Geometry check sheet. Reference: the model listing, model coordinates, mm. Give positions to 0.01 mm unless a question says otherwise; leave off trailing zeros. Loops run counter-clockwise (first coordinate to the right, second up) from the corner with the lowest first, then second, coordinate; pieces in that order, holes last. Notation, with made-up numbers: (45.5, -12.5) -> (79.5, -12.5) arc R20 cw to (79.5, 19.5) -> close; hole circle Ø7 at (33.5, 83). An arc over 180 degrees is marked (long way). Write item = value, one per line. Start each with the question number.
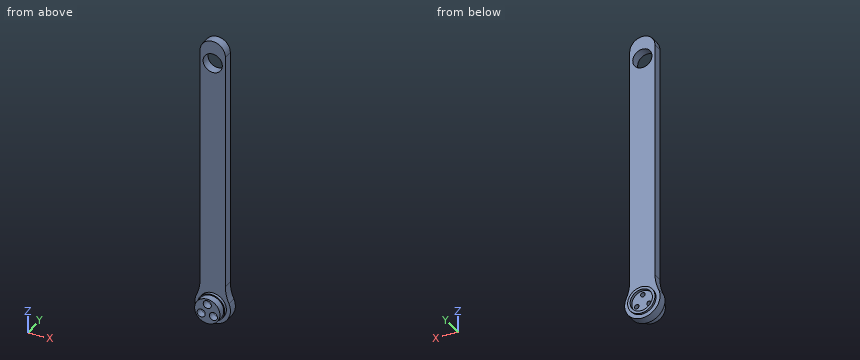
```python
from build123d import *
from build123d.topology import SkipClean

# Parameters (mm, degrees)
EXTRUDE_1_DEPTH              = 9
SKETCH_3_R                   = 13.5
EXTRUDE_2_DEPTH              = 2
SKETCH_4_R                   = 13.5
EXTRUDE_3_DEPTH              = 3
SKETCH_5_R                   = 9.5
CUT_EXTRUDE_2_DEPTH          = 274.324898244
HOLE_WIZARD_M4_1_D           = 4.5
HOLE_WIZARD_M4_1_CBORE_D     = 8
HOLE_WIZARD_M4_1_CBORE_DEPTH = 4.4
PATTERN_CIRCULAR_1_COUNT     = 3
SKETCH_11_R                  = 12.5
SKETCH_11_R_2                = 4
EXTRUDE_4_DEPTH              = 7
SKETCH_13_R                  = 11
CUT_EXTRUDE_3_DEPTH          = 3
FILLET_1_R                   = 40


with BuildPart() as part:
    # Sketch 1 → Extrude 1 (new body)
    with BuildSketch(Plane(origin=(0, 0, 0), x_dir=(1, 0, 0), z_dir=(0, 1, 0))):
        with BuildLine():
            Line((-12.5, -260), (-12.5, -12.247448714))
            ThreePointArc((-12.5, -12.247448714), (0, 17.5), (12.5, -12.247448714))
            Line((12.5, -12.247448714), (12.5, -260))
            ThreePointArc((12.5, -260), (0, -272.5), (-12.5, -260))
        make_face()
    extrude(amount=EXTRUDE_1_DEPTH)

    # Sketch 3 → Extrude 2 (add)
    with BuildSketch(Plane(origin=(0, 9, 0), x_dir=(1, 0, 0), z_dir=(0, 1, 0))):
        with Locations(Location((0, 0, 0), (0, 0, 270))):
            Circle(SKETCH_3_R)
    extrude(amount=EXTRUDE_2_DEPTH)

    # Sketch 4 → Extrude 3 (add)
    with BuildSketch(Plane.XZ):
        with Locations(Location((0, 0, 0), (0, 0, 90))):
            Circle(SKETCH_4_R)
    extrude(amount=EXTRUDE_3_DEPTH)

    # Sketch 5 → Cut-Extrude 2 (cut, through all)
    with BuildSketch(Plane(origin=(0, 9, 0), x_dir=(1, 0, 0), z_dir=(0, 1, 0))):
        with Locations(Location((0, -250, 0), (0, 0, 270))):
            Circle(SKETCH_5_R)
    extrude(amount=-CUT_EXTRUDE_2_DEPTH, mode=Mode.SUBTRACT)

    # Hole Wizard M4 _ _ _ _ _ _1 (through all)
    with Locations(Plane(origin=(0, -3, 0), x_dir=(-1, 0, 0), z_dir=(0, -1, 0))):
        with Locations((0, -7)):
            hole_wizard_m4_1 = CounterBoreHole(HOLE_WIZARD_M4_1_D / 2, HOLE_WIZARD_M4_1_CBORE_D / 2, HOLE_WIZARD_M4_1_CBORE_DEPTH)

    # Pattern Circular 1: Hole Wizard M4 _ _ _ _ _ _1 ×3 about axis
    pattern_circular_1_axis = Axis((0, 0, 0), (0, 1, 0))
    for i in range(1, PATTERN_CIRCULAR_1_COUNT):
        add(hole_wizard_m4_1.rotate(pattern_circular_1_axis, i * 360 / PATTERN_CIRCULAR_1_COUNT), mode=Mode.SUBTRACT)

    # Sketch 11 → Extrude 4 (add)
    with SkipClean():  # the faces are left unmerged after this step: merging them gives an invalid solid
        with BuildSketch(Plane.XZ.offset(3)):
            with Locations(Location((0, 0, 0), (0, 0, 270))):
                Circle(SKETCH_11_R)
            with Locations(Location((6.062177826, -3.5, 0), (0, 0, 270))):
                Circle(SKETCH_11_R_2, mode=Mode.SUBTRACT)
            with Locations(Location((0, 7, 0), (0, 0, 270))):
                Circle(SKETCH_11_R_2, mode=Mode.SUBTRACT)
            with Locations(Location((-6.062177826, -3.5, 0), (0, 0, 270))):
                Circle(SKETCH_11_R_2, mode=Mode.SUBTRACT)
        extrude(amount=EXTRUDE_4_DEPTH)

    # Sketch 13 → Cut-Extrude 3 (cut)
    with SkipClean():  # the faces are left unmerged after this step: merging them gives an invalid solid
        with BuildSketch(Plane(origin=(0, 11, 0), x_dir=(1, 0, 0), z_dir=(0, 1, 0))):
            with Locations(Location((0, 0, 0), (0, 0, 270))):
                Circle(SKETCH_13_R)
        extrude(amount=-CUT_EXTRUDE_3_DEPTH, mode=Mode.SUBTRACT)

    # Fillet 1
    fillet_1_edges = [part.edges().sort_by_distance(p)[0] for p in [
        (12.5, 4.5, 12.247448714),
        (-12.5, 4.5, 12.247448714),
    ]]
    fillet(fillet_1_edges, radius=FILLET_1_R)


solid = part.part
```
1) Thickness scan on line 1 (Z direction, x = -0.5, y = 0.5); line 2 (Z direction, x = -6.5, y = 1.75); line 3 (X direction, y = -5.25, z = -3.5). Record the ranges inside material, lowest first.
2) Depth check by flat-ended pin: pin 1 Ø2.5 at (x, z) = (8, -3) entering from -Y; pin 2 Ø3.5 at (x, z) = (6.06, -3.5) entering from +Y; pin 3 Ø10.5 at (x, z) = (6.5, 111.5) entering from +Y; pin 4 Ø4 at (y, z) = (6, 80.5) entering from +X. Enter the tip coordinate at first touch or a pass-through.
3) Section check A-A (z = 106.5). Enter the section's corners in (x, y), plus the area to 3 significant figures.
Check result:
q1.line_1 = -17.49 to 3.03, 10.97 to 240.51, 259.49 to 272.49
q1.line_2 = -16.25 to -5.71, -1.29 to 243.07, 256.93 to 270.68
q1.line_3 = -12 to -10.06, -2.06 to 2.06, 10.06 to 12
q2.pin_1 = 1.4
q2.pin_2 = through
q2.pin_3 = 9
q2.pin_4 = 12.5
q3.outline = (-12.5, 0) -> (12.5, 0) -> (12.5, 9) -> (-12.5, 9) -> close
q3.area = 225 mm2
